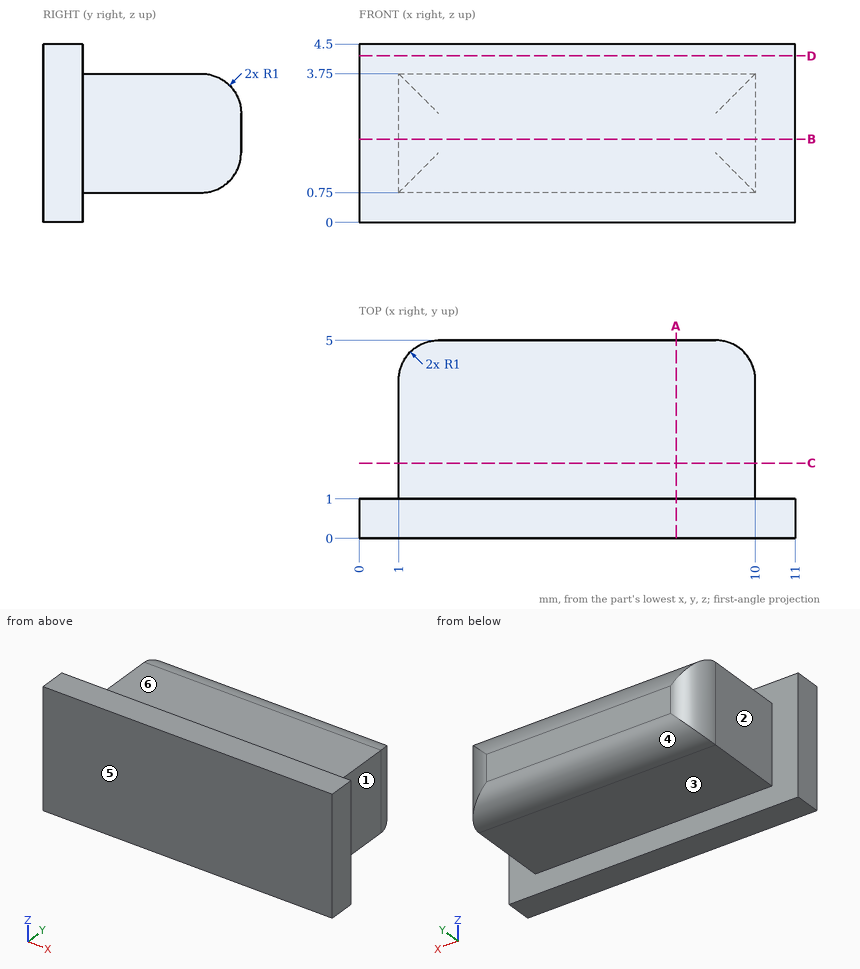
The figure shows three views and two pictorial views of one solid part (mm, origin at its lowest corner). Answer the questions. A direction names the side the tool comes from. Round coordinates to 2 decimals unless told otherwise and drop trailing zeros. Loops run counter-clockwise (first coordinate to the right, second up) from the corner with the lowest first, then second, coordinate; pieces in that order, holes last. Notation, with made-up numbers: (15, 81.5) - (19, 81.5) arc R27 ccw to (19, 98.5) - close; hole circle Ø5 at (14.5, 11.25). An arc over 180 degrees is marked (long way). One line per question, with ' | ' between items. Start each with the question number.
Q1. Section B-B on z = 2.1 is taken. Give the vertices of the cut face in (x, y), plus the area to 3 significant figures.
Q2. Section C-C on y = 1.9 is taken. Give the vertices of the cut face in (x, z).
Q3. Section D-D on z = 4.2 is taken. Give the vertices of the cut face in (x, y).
Q4. Find the intervals of material crossed by L1, parallel to X at y = 3.1, z = 2.75; L2, parallel to Z at x = 9.75, y = 3.9; L3, parallel to Y at x = 2.75, z = 4.25, in increasing order.
Q5. Flat-ended cylindrical pins translate along their axes: pin 1 (1.5 mm diameter, centred on x = 7.5, y = 2, fed in from -Z); pin 2 (0.9 mm diameter, centred on y = 2, z = 2.5, fed in from -X); pin 3 (2.5 mm diameter, centred on x = 6, y = 2.5, fed in from +Z). Find the tip coordinate at first contact, or state that the pin passes through.
Q6. Section A-A on x = 8 is taken. Give the vertices of the cut face in (y, z).
Q7. For a pull along Z with two mould halves and no side action, classify the marked faces 4, 5 and 6 as +Z half, -Z half, draft (parallel to the pull), parting line (faces both ways), or undercut.
Q8. For the marked faces 1, 2 and 3, determine the directions among +Z, -Z, +X, -X, +Y, -Y from which every point of the face is accessible in a straight line to the end or side of a thin tool.
Established:
1) outline: (0, 0) - (11, 0) - (11, 1) - (10, 1) - (10, 4) arc R1 ccw to (9, 5) - (2, 5) arc R1 ccw to (1, 4) - (1, 1) - (0, 1) - close | area: 46.6 mm²
2) outline: (1, 0.75) - (10, 0.75) - (10, 3.75) - (1, 3.75) - close
3) outline: (0, 0) - (11, 0) - (11, 1) - (0, 1) - close
4) L1: 1 to 10 | L2: 0.75 to 3.75 | L3: 0 to 1
5) pin 1: z = 0.75 | pin 2: x = 1 | pin 3: z = 3.75
6) outline: (0, 0) - (1, 0) - (1, 0.75) - (4, 0.75) arc R1 ccw to (5, 1.75) - (5, 2.75) arc R1 ccw to (4, 3.75) - (1, 3.75) - (1, 4.5) - (0, 4.5) - close
7) face 4: -Z half | face 5: draft | face 6: +Z half
8) face 1: +Z, -Z, +X, +Y | face 2: +Z, -Z, -X, +Y | face 3: -Z, +X, -X, +Y
